```python
from build123d import *

# Parameters (mm, degrees)
SKETCH_181_R      = 2.5
EXTRUDE_724_DEPTH = 250


with BuildPart() as part:
    # Sketch 181 → Extrude 724 (new body)
    with BuildSketch(Plane.XY):
        with BuildLine():
            Line((-4, 1.898780669), (-4, 0.337695265))
            ThreePointArc((-4, 0.337695265), (-3.98590708, 0.254943529), (-3.945217202, 0.181521503))
            Line((-3.945217202, 0.181521503), (-3.8, 0))
            Line((-3.8, 0), (-3.945217202, -0.181521503))
            ThreePointArc((-3.945217202, -0.181521503), (-3.98590708, -0.254943529), (-4, -0.337695265))
            Line((-4, -0.337695265), (-4, -1.898780669))
            ThreePointArc((-4, -1.898780669), (-4.152240935, -2.664147534), (-4.585786438, -3.312994231))
            Line((-4.585786438, -3.312994231), (-6.279898987, -5.007106781))
            ThreePointArc((-6.279898987, -5.007106781), (-6.604322336, -5.223879533), (-6.987005769, -5.3))
            Line((-6.987005769, -5.3), (-7.8, -5.3))
            ThreePointArc((-7.8, -5.3), (-7.941421356, -5.241421356), (-8, -5.1))
            Line((-8, -5.1), (-8, -3.33))
            ThreePointArc((-8, -3.33), (-8.154329142, -3.099030117), (-8.426776695, -3.153223305))
            Line((-8.426776695, -3.153223305), (-9.926776695, -4.653223305))
            ThreePointArc((-9.926776695, -4.653223305), (-9.980969883, -4.734329142), (-10, -4.83))
            Line((-10, -4.83), (-10, -8.5))
            ThreePointArc((-10, -8.5), (-9.560660172, -9.560660172), (-8.5, -10))
            Line((-8.5, -10), (-4.83, -10))
            ThreePointArc((-4.83, -10), (-4.734329142, -9.980969883), (-4.653223305, -9.926776695))
            Line((-4.653223305, -9.926776695), (-3.153223305, -8.426776695))
            ThreePointArc((-3.153223305, -8.426776695), (-3.099030117, -8.154329142), (-3.33, -8))
            Line((-3.33, -8), (-5.1, -8))
            ThreePointArc((-5.1, -8), (-5.241421356, -7.941421356), (-5.3, -7.8))
            Line((-5.3, -7.8), (-5.3, -6.987005769))
            ThreePointArc((-5.3, -6.987005769), (-5.223879533, -6.604322336), (-5.007106781, -6.279898987))
            Line((-5.007106781, -6.279898987), (-3.312994231, -4.585786438))
            ThreePointArc((-3.312994231, -4.585786438), (-2.664147534, -4.152240935), (-1.898780669, -4))
            Line((-1.898780669, -4), (-0.337695265, -4))
            ThreePointArc((-0.337695265, -4), (-0.254943529, -3.98590708), (-0.181521503, -3.945217202))
            Line((-0.181521503, -3.945217202), (0, -3.8))
            Line((0, -3.8), (0.181521503, -3.945217202))
            ThreePointArc((0.181521503, -3.945217202), (0.254943529, -3.98590708), (0.337695265, -4))
            Line((0.337695265, -4), (1.898780669, -4))
            ThreePointArc((1.898780669, -4), (2.664147534, -4.152240935), (3.312994231, -4.585786438))
            Line((3.312994231, -4.585786438), (5.007106781, -6.279898987))
            ThreePointArc((5.007106781, -6.279898987), (5.223879533, -6.604322336), (5.3, -6.987005769))
            Line((5.3, -6.987005769), (5.3, -7.8))
            ThreePointArc((5.3, -7.8), (5.241421356, -7.941421356), (5.1, -8))
            Line((5.1, -8), (3.33, -8))
            ThreePointArc((3.33, -8), (3.099030117, -8.154329142), (3.153223305, -8.426776695))
            Line((3.153223305, -8.426776695), (4.653223305, -9.926776695))
            ThreePointArc((4.653223305, -9.926776695), (4.734329142, -9.980969883), (4.83, -10))
            Line((4.83, -10), (8.5, -10))
            ThreePointArc((8.5, -10), (9.560660172, -9.560660172), (10, -8.5))
            Line((10, -8.5), (10, -4.83))
            ThreePointArc((10, -4.83), (9.980969883, -4.734329142), (9.926776695, -4.653223305))
            Line((9.926776695, -4.653223305), (8.426776695, -3.153223305))
            ThreePointArc((8.426776695, -3.153223305), (8.154329142, -3.099030117), (8, -3.33))
            Line((8, -3.33), (8, -5.1))
            ThreePointArc((8, -5.1), (7.941421356, -5.241421356), (7.8, -5.3))
            Line((7.8, -5.3), (6.987005769, -5.3))
            ThreePointArc((6.987005769, -5.3), (6.604322336, -5.223879533), (6.279898987, -5.007106781))
            Line((6.279898987, -5.007106781), (4.585786438, -3.312994231))
            ThreePointArc((4.585786438, -3.312994231), (4.152240935, -2.664147534), (4, -1.898780669))
            Line((4, -1.898780669), (4, -0.337695265))
            ThreePointArc((4, -0.337695265), (3.98590708, -0.254943529), (3.945217202, -0.181521503))
            Line((3.945217202, -0.181521503), (3.8, 0))
            Line((3.8, 0), (3.945217202, 0.181521503))
            ThreePointArc((3.945217202, 0.181521503), (3.98590708, 0.254943529), (4, 0.337695265))
            Line((4, 0.337695265), (4, 1.898780669))
            ThreePointArc((4, 1.898780669), (4.152240935, 2.664147534), (4.585786438, 3.312994231))
            Line((4.585786438, 3.312994231), (6.279898987, 5.007106781))
            ThreePointArc((6.279898987, 5.007106781), (6.604322336, 5.223879533), (6.987005769, 5.3))
            Line((6.987005769, 5.3), (7.8, 5.3))
            ThreePointArc((7.8, 5.3), (7.941421356, 5.241421356), (8, 5.1))
            Line((8, 5.1), (8, 3.33))
            ThreePointArc((8, 3.33), (8.154329142, 3.099030117), (8.426776695, 3.153223305))
            Line((8.426776695, 3.153223305), (9.926776695, 4.653223305))
            ThreePointArc((9.926776695, 4.653223305), (9.980969883, 4.734329142), (10, 4.83))
            Line((10, 4.83), (10, 8.5))
            ThreePointArc((10, 8.5), (9.560660172, 9.560660172), (8.5, 10))
            Line((8.5, 10), (4.83, 10))
            ThreePointArc((4.83, 10), (4.734329142, 9.980969883), (4.653223305, 9.926776695))
            Line((4.653223305, 9.926776695), (3.153223305, 8.426776695))
            ThreePointArc((3.153223305, 8.426776695), (3.099030117, 8.154329142), (3.33, 8))
            Line((3.33, 8), (5.1, 8))
            ThreePointArc((5.1, 8), (5.241421356, 7.941421356), (5.3, 7.8))
            Line((5.3, 7.8), (5.3, 6.987005769))
            ThreePointArc((5.3, 6.987005769), (5.223879533, 6.604322336), (5.007106781, 6.279898987))
            Line((5.007106781, 6.279898987), (3.312994231, 4.585786438))
            ThreePointArc((3.312994231, 4.585786438), (2.664147534, 4.152240935), (1.898780669, 4))
            Line((1.898780669, 4), (0.337695265, 4))
            ThreePointArc((0.337695265, 4), (0.254943529, 3.98590708), (0.181521503, 3.945217202))
            Line((0.181521503, 3.945217202), (0, 3.8))
            Line((0, 3.8), (-0.181521503, 3.945217202))
            ThreePointArc((-0.181521503, 3.945217202), (-0.254943529, 3.98590708), (-0.337695265, 4))
            Line((-0.337695265, 4), (-1.898780669, 4))
            ThreePointArc((-1.898780669, 4), (-2.664147534, 4.152240935), (-3.312994231, 4.585786438))
            Line((-3.312994231, 4.585786438), (-5.007106781, 6.279898987))
            ThreePointArc((-5.007106781, 6.279898987), (-5.223879533, 6.604322336), (-5.3, 6.987005769))
            Line((-5.3, 6.987005769), (-5.3, 7.8))
            ThreePointArc((-5.3, 7.8), (-5.241421356, 7.941421356), (-5.1, 8))
            Line((-5.1, 8), (-3.33, 8))
            ThreePointArc((-3.33, 8), (-3.099030117, 8.154329142), (-3.153223305, 8.426776695))
            Line((-3.153223305, 8.426776695), (-4.653223305, 9.926776695))
            ThreePointArc((-4.653223305, 9.926776695), (-4.734329142, 9.980969883), (-4.83, 10))
            Line((-4.83, 10), (-8.5, 10))
            ThreePointArc((-8.5, 10), (-9.560660172, 9.560660172), (-10, 8.5))
            Line((-10, 8.5), (-10, 4.83))
            ThreePointArc((-10, 4.83), (-9.980969883, 4.734329142), (-9.926776695, 4.653223305))
            Line((-9.926776695, 4.653223305), (-8.426776695, 3.153223305))
            ThreePointArc((-8.426776695, 3.153223305), (-8.154329142, 3.099030117), (-8, 3.33))
            Line((-8, 3.33), (-8, 5.1))
            ThreePointArc((-8, 5.1), (-7.941421356, 5.241421356), (-7.8, 5.3))
            Line((-7.8, 5.3), (-6.987005769, 5.3))
            ThreePointArc((-6.987005769, 5.3), (-6.604322336, 5.223879533), (-6.279898987, 5.007106781))
            Line((-6.279898987, 5.007106781), (-4.585786438, 3.312994231))
            ThreePointArc((-4.585786438, 3.312994231), (-4.152240935, 2.664147534), (-4, 1.898780669))
        make_face()
        with Locations(Location((0, 0, 0), (0, 0, 180))):
            Circle(SKETCH_181_R, mode=Mode.SUBTRACT)
    extrude(amount=-EXTRUDE_724_DEPTH)


solid = part.part
```
Check sheet for the modelled part. Datum: model origin and axes. Units: mm. Coordinates: 2 decimals unless noted, no trailing zeros. Write item = value, one per line. Start each with the question number.
1) Go/stop test with flat-tipped pins: P1, Ø1.7, axis at x = -1, z = -92, coming from the -Y side; P2, Ø0.9, axis at y = -4.5, z = -132.5, coming from the +X side; P3, Ø0.5, axis at x = -1, z = -65.5, coming from the +Y side; P4, Ø0.5, axis at y = 4, z = -84, coming from the -X side. Record where each tip stops, or that it passes through.
2) Mould release check, pull along Y, two halves, no side actions. Record for faces 1 (the cylindrical face through (2.5, -0.1, -123.2)), 2 (the flat face through (2, 2, 0)): +Y half, -Y half, draft (parallel to the pull), parting line (faces both ways), or undercut.
3) Material ranges on L1, parallel to Y at x = 7.5, z = -21.5; L2, parallel to Y at x = 0, z = -96; L3, parallel to X at y = 8.25, z = -22, recorded low to high.
Ans:
q1.P1 = -4
q1.P2 = 10
q1.P3 = 4
q1.P4 = -9.52
q2.face_1 = undercut
q2.face_2 = draft
q3.L1 = -10 to -5.3, 5.3 to 10
q3.L2 = -3.8 to -2.5, 2.5 to 3.8
q3.L3 = -10 to -3.08, 3.08 to 10
